Read the model definition and answer for the solid it produces. Units are mm, in the model's axes. A direction names the side the tool comes from. Round coordinates to 2 decimals unless told otherwise and drop trailing zeros. Write each loop counter-clockwise with the first axis right and the second up, starting at its lowest first coordinate (ties: lowest second). Pieces come first, ordered by that corner, then holes.
from build123d import *

# Parameters (mm, degrees)
F0_R     = 12.5
F1_DEPTH = 57.5
F2_R     = 3.5
F3_DEPTH = 10
F5_R     = 1.5
F6_R     = 0.5


with BuildPart() as f1:
    # F0 (on Right) → F1 (new body, symmetric)
    with BuildSketch(Plane.YZ):
        Circle(F0_R)
    extrude(amount=F1_DEPTH, both=True)

    # F2 (on face) → F3 (join)
    with BuildSketch(Plane(origin=(-57.5, 0, 0), x_dir=(0, -1, 0), z_dir=(-1, 0, 0))):
        Circle(F2_R)
    extrude(amount=F3_DEPTH)

    # F4: F1 across plane


with BuildPart() as f1_1:
    add(f1.part)
    add(f1.part.mirror(Plane.YZ))

    # F5
    f5_edges = [f1_1.edges().sort_by_distance(p)[0] for p in [
        (-57.5, -12.5, 0),
        (57.5, -12.5, 0),
    ]]
    fillet(f5_edges, radius=F5_R)

    # F6
    f6_edges = [f1_1.edges().sort_by_distance(p)[0] for p in [
        (67.5, 3.5, 0),
        (-67.5, 3.5, 0),
    ]]
    fillet(f6_edges, radius=F6_R)


solid = f1_1.part
Q1. Straight lines are drawn through the part: probe 1 along X at (y, z) = (5.5, 3.25); probe 2 along Z at (x, y) = (-56.5, 5.75); probe 3 along Z at (x, y) = (20, -5.75). For each, find the intervals that lie inside material, in ascending order.
Verdict:
probe 1: x = -57.5 to 57.5
probe 2: z = -11 to 11
probe 3: z = -11.1 to 11.1
Q2. Flat-ended cylindrical pins translate along their axes: pin 1 Ø1 at (x, z) = (49.5, 4) entering from -Y; pin 2 Ø8 at (x, y) = (45, 6.5) entering from -Z; pin 3 Ø6 at (y, z) = (-8.5, -2) entering from +X. Find the tip coordinate at first contact, or state that the pin passes through.
Verdict:
pin 1: stops at y = -12
pin 2: stops at z = -12.25
pin 3: stops at x = 57.5
Q3. Section C-C (x = -50.5) is taken. Determine the outline of the cut face in (y, z).
Verdict:
outline: circle Ø25 at (0, 0)
Q4. Section A-A (z = 0) is taken. Determine the outline of the cut face in (x, y).
Verdict:
outline: (-67.5, -3) arc R0.5 ccw to (-67, -3.5) - (-57.5, -3.5) - (-57.5, -11) arc R1.5 ccw to (-56, -12.5) - (56, -12.5) arc R1.5 ccw to (57.5, -11) - (57.5, -3.5) - (67, -3.5) arc R0.5 ccw to (67.5, -3) - (67.5, 3) arc R0.5 ccw to (67, 3.5) - (57.5, 3.5) - (57.5, 11) arc R1.5 ccw to (56, 12.5) - (-56, 12.5) arc R1.5 ccw to (-57.5, 11) - (-57.5, 3.5) - (-67, 3.5) arc R0.5 ccw to (-67.5, 3) - close
Q5. Which of the six approach directions +Z, -Z, +X, -X, +Y, -Y give full straight-line access (tool end or side, diameter ignored) to faces 1 (the cylindrical face through (62.184, -3.233, -1.341)), 2 (the flat face through (-67.5, 0, 0)), 3 (the flat face through (-57.5, -3, 3))?
Verdict:
face 1: +X
face 2: +Z, -Z, -X, +Y, -Y
face 3: -X
